Check sheet for the modelled part. Datum: model origin and axes. Units: mm. Face numbers are marked on the shaded views. A direction names the side the tool comes from. Give positions to 0.01 mm unless a question says otherwise; leave off trailing zeros. Loops run counter-clockwise (first coordinate to the right, second up) from the corner with the lowest first, then second, coordinate; pieces in that order, holes last. Notation, with made-up numbers: (2.5, 61.25) -> (61.5, 61.25) arc R23 cw to (61.5, 91.25) -> close; hole circle Ø7 at (0.25, 59). An arc over 180 degrees is marked (long way). Write each question's results on one line, items separated by ' | '. Start each with the question number.
Item 1: Mould release check, pull along X, two halves, no side actions. Record for the marked faces 3, 4 and 5: pulls with the +X half, pulls with the -X half, needs draft (parallel to the pull), parting line crosses it, or undercut.
Item 2: Cross-section at D-D on z = -4.5. Enter the section's corners in (x, y), then the cut area to 3 significant figures.
Item 3: Cross-section at A-A on z = 0. Enter the section's corners in (x, y).
Item 4: Gauge pin test, flat ends, axial feed: pin 1 Ø1 at (x, y) = (-3, 5) entering from +Z; pin 2 Ø3 at (y, z) = (1.5, 8.5) entering from +X; pin 3 Ø1 at (x, y) = (-12.5, 1.5) entering from -Z; pin 4 Ø3 at (x, z) = (8, 0) entering from -Y. Record the tip position at first contact, or that the pin passes through.
Item 5: Access from +Z, -Z, +X, -X, +Y, -Y to the whole of each face (thin tool, end or side, straight path). Record for the marked faces 1 and 2.
Item 6: Cross-section at C-C on x = 12.5. Enter the section's corners in (y, z), then the cut area to 3 significant figures.
Item 7: Cross-section at B-B on y = 0.45. Enter the section's corners in (x, z), then the cut area to 3 significant figures.
Item 8: Scan lines: line 1 along X through (y, z) = (0.5, 0); line 2 along X through (y, z) = (1.5, 8); line 3 along Y through (x, z) = (12.5, 1.25). Record each from-to range of solid material in increasing order.
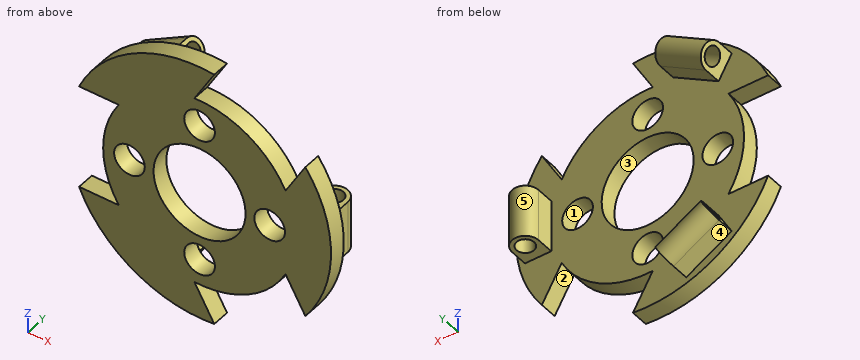
from build123d import *

# Parameters (mm, degrees)
SKETCH1_R           = 15
SKETCH1_R_2         = 5.25
SKETCH1_R_3         = 1.75
BOSS_EXTRUDE1_DEPTH = 2
SKETCH2_R           = 1
BOSS_EXTRUDE2_DEPTH = 3
CIRPATTERN1_COUNT   = 3
SKETCH3_OUTSIDE_W   = 40.556
SKETCH3_OUTSIDE_H   = 40.556
CUT_EXTRUDE1_DEPTH  = 10


with BuildPart() as part:
    # Sketch1 → Boss-Extrude1 (new body)
    with BuildSketch(Plane(origin=(0, 0, 0), x_dir=(1, 0, 0), z_dir=(0, 1, 0))):
        with Locations(Location((0, 0, 0), (0, 0, 270))):
            Circle(SKETCH1_R)
        with Locations(Location((0, 0, 0), (0, 0, 270))):
            Circle(SKETCH1_R_2, mode=Mode.SUBTRACT)
        with Locations(Location((0, 8, 0), (0, 0, 270))):
            Circle(SKETCH1_R_3, mode=Mode.SUBTRACT)
        with Locations(Location((8, 0, 0), (0, 0, 270))):
            Circle(SKETCH1_R_3, mode=Mode.SUBTRACT)
        with Locations(Location((0, -8, 0), (0, 0, 270))):
            Circle(SKETCH1_R_3, mode=Mode.SUBTRACT)
        with Locations(Location((-8, 0, 0), (0, 0, 270))):
            Circle(SKETCH1_R_3, mode=Mode.SUBTRACT)
    extrude(amount=BOSS_EXTRUDE1_DEPTH)

    # Sketch2 → Boss-Extrude2 (add, symmetric)
    with BuildSketch(Plane.XY):
        with BuildLine():
            Line((11, 2), (11, 4))
            ThreePointArc((11, 4), (12.5, 5.5), (14, 4))
            Line((14, 4), (14, 2))
            Line((14, 2), (11, 2))
        make_face()
        with Locations((12.5, 4)):
            Circle(SKETCH2_R, mode=Mode.SUBTRACT)
    boss_extrude2 = extrude(amount=BOSS_EXTRUDE2_DEPTH, both=True)

    # CirPattern1: Boss-Extrude2 ×3 about axis
    cirpattern1_axis = Axis((0, 0, 0), (0, 1, 0))
    for i in range(1, CIRPATTERN1_COUNT):
        add(boss_extrude2.rotate(cirpattern1_axis, i * 360 / CIRPATTERN1_COUNT))

    # Sketch3 outside → Cut-Extrude1 (cut)
    with BuildSketch(Plane(origin=(0, 2, 0), x_dir=(1, 0, 0), z_dir=(0, 1, 0))):
        Rectangle(SKETCH3_OUTSIDE_W, SKETCH3_OUTSIDE_H)
        with BuildLine():
            Line((1.67771112, -14.9058809), (-0.586380194, -10.984359711))
            ThreePointArc((-0.586380194, -10.984359711), (5.5, -9.526279442), (9.805924651, -4.984359711))
            Line((9.805924651, -4.984359711), (12.070015965, -8.9058809))
            ThreePointArc((12.070015965, -8.9058809), (15, 0), (12.070015965, 8.9058809))
            Line((12.070015965, 8.9058809), (9.805924651, 4.984359711))
            ThreePointArc((9.805924651, 4.984359711), (5.5, 9.526279442), (-0.586380194, 10.984359711))
            Line((-0.586380194, 10.984359711), (1.67771112, 14.9058809))
            ThreePointArc((1.67771112, 14.9058809), (-7.5, 12.990381057), (-13.747727085, 6))
            Line((-13.747727085, 6), (-9.219544457, 6))
            ThreePointArc((-9.219544457, 6), (-11, 0), (-9.219544457, -6))
            Line((-9.219544457, -6), (-13.747727085, -6))
            ThreePointArc((-13.747727085, -6), (-7.5, -12.990381057), (1.67771112, -14.9058809))
        make_face(mode=Mode.SUBTRACT)
    extrude(amount=-CUT_EXTRUDE1_DEPTH, mode=Mode.SUBTRACT)


solid = part.part
Answer sheet:
1) face 3: undercut | face 4: pulls with the -X half | face 5: parting line crosses it
2) outline: (-10.04, 0) -> (-2.7, 0) -> (-2.7, 2) -> (-10.04, 2) -> close; (2.7, 0) -> (14.31, 0) -> (14.31, 2) -> (2.7, 2) -> close | area: 37.9 mm²
3) outline: (-11, 0) -> (-9.75, 0) -> (-9.75, 2) -> (-11, 2) -> close; (-6.25, 0) -> (-5.25, 0) -> (-5.25, 2) -> (-6.25, 2) -> close; (5.25, 0) -> (6.25, 0) -> (6.25, 2) -> (5.25, 2) -> close; (9.75, 0) -> (15, 0) -> (15, 2) -> (14, 2) -> (14, 4) arc R1.5 ccw to (11, 4) -> (11, 2) -> (9.75, 2) -> close; hole circle Ø2 at (12.5, 4)
4) pin 1: stops at z = 12.06 | pin 2: stops at x = 13.27 | pin 3: stops at z = -9 | pin 4: passes through
5) face 1: +Y, -Y | face 2: -Z, +Y, -Y
6) outline: (0, -8.29) -> (2, -8.29) -> (2, -3) -> (3, -3) -> (3, 3) -> (2, 3) -> (2, 8.29) -> (0, 8.29) -> close; (5, -3) -> (5.5, -3) -> (5.5, 3) -> (5, 3) -> close | area: 42.2 mm²
7) outline: (-13.75, -6) arc R15 ccw to (1.68, -14.91) -> (-0.59, -10.98) arc R11 ccw to (9.81, -4.98) -> (12.07, -8.91) arc R15 ccw to (12.07, 8.91) -> (9.81, 4.98) arc R11 ccw to (-0.59, 10.98) -> (1.68, 14.91) arc R15 ccw to (-13.75, 6) -> (-9.22, 6) arc R11 ccw to (-9.22, -6) -> close; hole circle Ø3.5 at (-8, 0); hole circle Ø10.5 at (0, 0); hole circle Ø3.5 at (0, -8); hole circle Ø3.5 at (0, 8); hole circle Ø3.5 at (8, 0) | area: 432 mm²
8) line 1: x = -11 to -9.75, -6.25 to -5.25, 5.25 to 6.25, 9.75 to 15 | line 2: x = -12.69 to -1.75, 1.75 to 7.55, 11.55 to 12.69 | line 3: y = 0 to 3, 5 to 5.5
